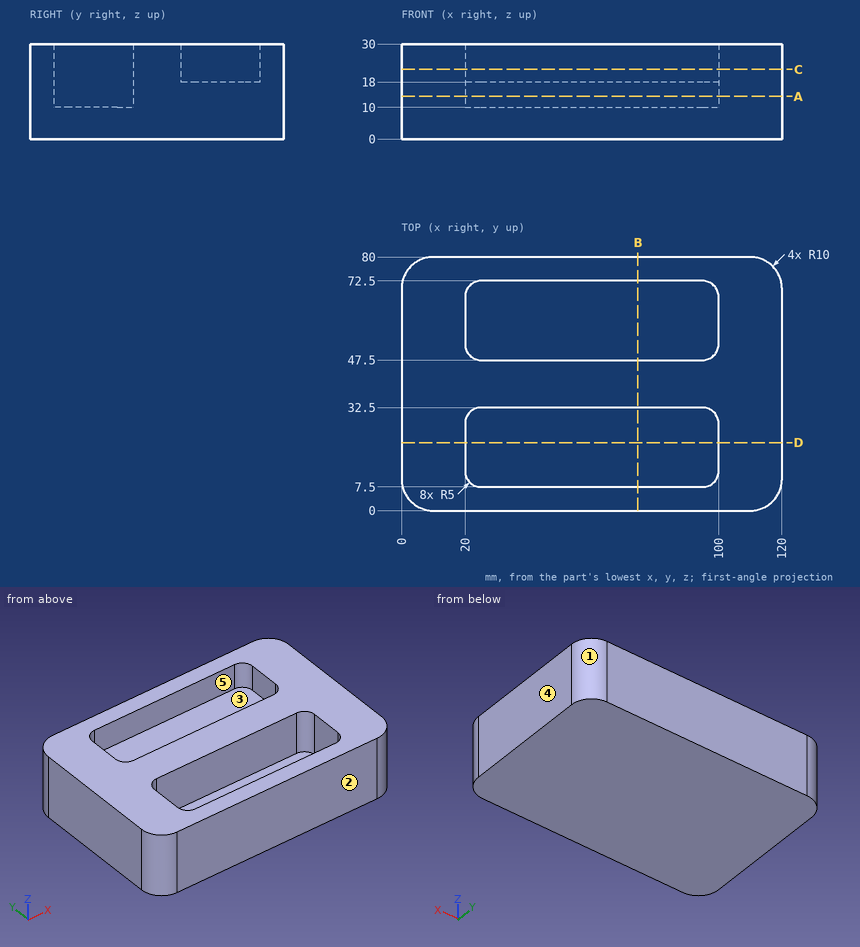
For this review, use the dimensioned drawing (mm, ordinates from the lowest corner) and the shaded views. A direction names the side the tool comes from. Coordinates: 2 decimals unless noted, no trailing zeros. Order: outer loops, then holes, each group sorted by start corner. A loop starts at its lowest first (then second) coordinate and runs counter-clockwise, first axis right, second up. Notation, with made-up numbers: M 85,-1 L 91,-1 A19 cw 91,26 Z; hole C -12,-17.5 d11. An arc over 180 degrees is marked long. Answer as a JSON object with one key per item and string values. Group by question number.
1) Tool access review of the marked faces 4 and 5: name each direction out of +Z, -Z, +X, -X, +Y, -Y from which nothing blocks a thin tool from reaching the whole face with its end or side.
2) Wall thickness on L1, parallel to Y at x = 68, z = 22.25; L2, parallel to X at y = 21.5, z = 17; L3, parallel to Y at x = 73.5, z = 16.5: over which ranges is each line inside the solid? List them lowest first.
3) Add section B-B, the plane x = 74.5. Write out the cut boundary in (y, z), then the cut area to 3 significant figures.
4) Mouldability with a two-part tool opening along Y and no side actions: class the marked faces 1, 2 and 3 as pulls with the +Y half, pulls with the -Y half, needs draft (parallel to the pull), parting line crosses it, or undercut.
5) Add section D-D, the plane y = 21.5. Write out the cut boundary in (x, z), then the cut area to 3 significant figures.
6) Add section C-C, the plane z = 22. Write out the cut boundary in (x, y), then the cut area to 3 significant figures.
7) For pin 1 (5 mm diameter, centred on x = 69, y = 47, fed in from -Z); pin 2 (20 mm diameter, centred on x = 75.5, y = 60.5, fed in from +Z), all flat-tipped, find the tip position at first contact; note any pin that passes through.
8) Add section A-A, the plane z = 13.5. Write out the cut boundary in (x, y), then the cut area to 3 significant figures.
Computed values:
{
 "1": {"face 4": "+Z, -Z, +X, +Y, -Y", "face 5": "+Z"},
 "2": {"L1": "y = 0 to 7.5, 32.5 to 47.5, 72.5 to 80", "L2": "x = 0 to 20, 100 to 120", "L3": "y = 0 to 7.5, 32.5 to 80"},
 "3": {"outline": "M 0,0 L 80,0 L 80,30 L 72.5,30 L 72.5,18 L 47.5,18 L 47.5,30 L 32.5,30 L 32.5,10 L 7.5,10 L 7.5,30 L 0,30 Z", "area": "1,600 mm^2"},
 "4": {"face 1": "pulls with the +Y half", "face 2": "pulls with the -Y half", "face 3": "undercut"},
 "5": {"outline": "M 0,0 L 120,0 L 120,30 L 100,30 L 100,10 L 20,10 L 20,30 L 0,30 Z", "area": "2,000 mm^2"},
 "6": {"outline": "M 0,10 A10 ccw 10,0 L 110,0 A10 ccw 120,10 L 120,70 A10 ccw 110,80 L 10,80 A10 ccw 0,70 Z; hole M 20,12.5 A5 ccw 25,7.5 L 95,7.5 A5 ccw 100,12.5 L 100,27.5 A5 ccw 95,32.5 L 25,32.5 A5 ccw 20,27.5 Z; hole M 20,52.5 A5 ccw 25,47.5 L 95,47.5 A5 ccw 100,52.5 L 100,67.5 A5 ccw 95,72.5 L 25,72.5 A5 ccw 20,67.5 Z", "area": "5,560 mm^2"},
 "7": {"pin 1": "stops at z = 0", "pin 2": "stops at z = 18"},
 "8": {"outline": "M 0,10 A10 ccw 10,0 L 110,0 A10 ccw 120,10 L 120,70 A10 ccw 110,80 L 10,80 A10 ccw 0,70 Z; hole M 20,12.5 A5 ccw 25,7.5 L 95,7.5 A5 ccw 100,12.5 L 100,27.5 A5 ccw 95,32.5 L 25,32.5 A5 ccw 20,27.5 Z", "area": "7,540 mm^2"}
}
